Part model, mm, in its own coordinate system. Face numbers are marked on the shaded views. A direction names the side the tool comes from. Give positions to 0.01 mm unless a question says otherwise; leave off trailing zeros. Order: outer loops, then holes, each group sorted by start corner. A loop starts at its lowest first (then second) coordinate and runs counter-clockwise, first axis right, second up. Notation, with made-up numbers: (89.25, 20.5) -> (101.25, 20.5) arc R20 ccw to (101.25, 31.5) -> close; hole circle Ø2 at (30.25, 12). An arc over 180 degrees is marked (long way). Write item = value, one per line. Start each with the question number.
Item 1: Flat gauge pins, fed straight in: P1, Ø3, axis at x = -10, z = -3.5, coming from the -Y side; P2, Ø0.9, axis at y = 47, z = 1, coming from the -X side; P3, Ø1.5, axis at y = 48, z = -0.5, coming from the +X side; P4, Ø6, axis at x = -1, z = 4.5, coming from the +Y side. Where does each tip first touch, or does it go through?
Item 2: Band-saw the part on B-B on x = 7. Write the cut outline in (y, z).
Item 3: Drill centre lines: line 1 along X through (y, z) = (47.15, 0) (3 decimals); line 2 along Y through (x, z) = (3.25, 5); line 3 along X through (y, z) = (28, 7.5). Where is each one in solid material? Low to high.
Item 4: Band-saw the part on A-A on z = 0. Write the cut outline in (x, y) (3 decimals).
Item 5: Tool access for the marked faces 1 and 2: list every direction of +Z, -Z, +X, -X, +Y, -Y with a clear straight run to the whole face (end or side of a thin tool).
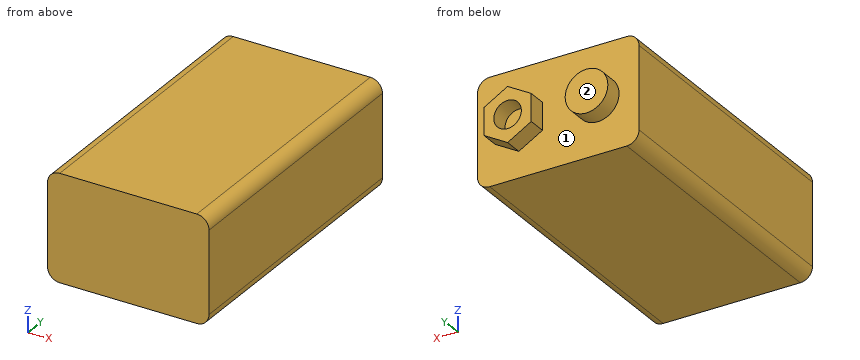
```python
from build123d import *

# Parameters (mm, degrees)
BOSS_EXTRUDE1_DEPTH = 46.4
SKETCH2_R           = 3.5
SKETCH2_R_2         = 2.259315118
BOSS_EXTRUDE2_DEPTH = 3


with BuildPart() as part:
    # Sketch1 → Boss-Extrude1 (new body)
    with BuildSketch(Plane(origin=(0, 0, 0), x_dir=(1, 0, 0), z_dir=(0, 1, 0))):
        with BuildLine():
            Line((-11.25, -8.75), (11.25, -8.75))
            ThreePointArc((11.25, -8.75), (12.664213562, -8.164213562), (13.25, -6.75))
            Line((13.25, -6.75), (13.25, 6.75))
            ThreePointArc((13.25, 6.75), (12.664213562, 8.164213562), (11.25, 8.75))
            Line((11.25, 8.75), (-11.25, 8.75))
            ThreePointArc((-11.25, 8.75), (-12.664213562, 8.164213562), (-13.25, 6.75))
            Line((-13.25, 6.75), (-13.25, -6.75))
            ThreePointArc((-13.25, -6.75), (-12.664213562, -8.164213562), (-11.25, -8.75))
        make_face()
    extrude(amount=BOSS_EXTRUDE1_DEPTH)

    # Sketch2 → Boss-Extrude2 (add)
    # profile 1 of 2: a face of its own
    with BuildSketch(Plane(origin=(0, 46.4, 0), x_dir=(1, 0, 0), z_dir=(0, 1, 0))):
        with Locations(Location((-6.475, 0, 0), (0, 0, 270))):
            Circle(SKETCH2_R)
    # profile 2 of 2: a face of its own
    with BuildSketch(Plane(origin=(0, 46.4, 0), x_dir=(1, 0, 0), z_dir=(0, 1, 0))):
        Polygon((6.475, 4.48194599), (2.593520914, 2.240972995), (2.593520914, -2.240972995), (6.475, -4.48194599), (10.356479086, -2.240972995), (10.356479086, 2.240972995), align=None)
        with Locations(Location((6.475, 0, 0), (0, 0, 270))):
            Circle(SKETCH2_R_2, mode=Mode.SUBTRACT)
    extrude(amount=BOSS_EXTRUDE2_DEPTH)


solid = part.part
```
Values found:
q1.P1 = 0
q1.P2 = -9.93
q1.P3 = 10.36
q1.P4 = 46.4
q2.outline = (0, -8.75) -> (46.4, -8.75) -> (46.4, -4.18) -> (49.4, -4.18) -> (49.4, -2.2) -> (46.4, -2.2) -> (46.4, 2.2) -> (49.4, 2.2) -> (49.4, 4.18) -> (46.4, 4.18) -> (46.4, 8.75) -> (0, 8.75) -> close
q3.line_1 = -9.975 to -2.975, 2.594 to 4.216, 8.734 to 10.356
q3.line_2 = 0 to 46.4
q3.line_3 = -13.1 to 13.1
q4.outline = (-13.25, 0) -> (13.25, 0) -> (13.25, 46.4) -> (10.356, 46.4) -> (10.356, 49.4) -> (8.734, 49.4) -> (8.734, 46.4) -> (4.216, 46.4) -> (4.216, 49.4) -> (2.594, 49.4) -> (2.594, 46.4) -> (-2.975, 46.4) -> (-2.975, 49.4) -> (-9.975, 49.4) -> (-9.975, 46.4) -> (-13.25, 46.4) -> close
q5.face_1 = +Y
q5.face_2 = +Z, -Z, +X, -X, +Y
